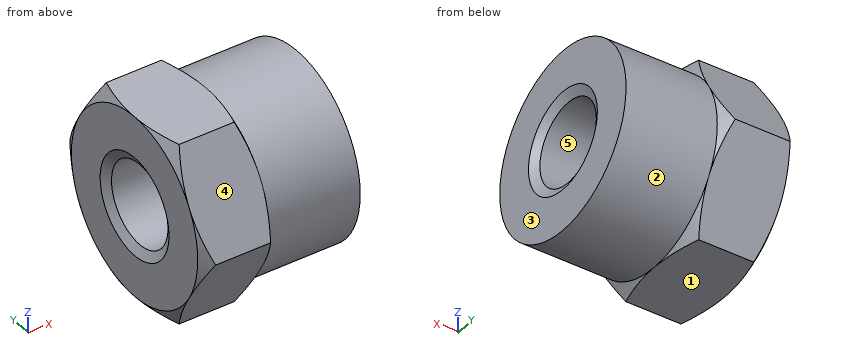
Autodesk Inventor part; units mm, degrees
ref_plane "Work Plane1" through (9.7259, 0, 0) normal (0, 0, 1) x (-1, 0, 0)
ref_plane "YZ Plane" through (0, 0, 0) normal (1, 0, 0) x (0, 1, 0)
ref_plane "XZ Plane" through (0, 0, 0) normal (0, 1, 0) x (-1, 0, 0)
sketch "Sketch1" plane through (0, 0, 0) normal (1, 0, 0) x (0, 1, 0)
  line L0 (1.5877, -2.75) -> (-1.5877, -2.75)
  line L1 (-1.5877, -2.75) -> (-3.1754, 0)
  line L2 (-3.1754, 0) -> (-1.5877, 2.75)
  line L3 (-1.5877, 2.75) -> (1.5877, 2.75)
  line L4 (1.5877, 2.75) -> (3.1754, 0)
  line L5 (3.1754, 0) -> (1.5877, -2.75)
  point P0 (0, 0)
  point P1 (0, 0)
  dimension "d0" = 6.3509
extrude "Body" add sketch "Sketch1" along normal blind 2.15
sketch "Sketch2" plane through (2.15, 0, 0) normal (1, 0, 0) x (0, 0, -1)
  circle A0 centre (0, 0) radius 2.75
  dimension "d7" = 5.5
extrude "Ring" add sketch "Sketch2" along normal blind 2.75
sketch "Sketch3" plane through (0, 0, 0) normal (0, 0, 1) x (1, 0, 0)
  line L0 (0, 1.5877) -> (0, 3.1754)
  line L1 (0, 3.1754) -> (2.15, 3.1754)
  line L2 (2.15, 1.5877) -> (2.15, 3.1754)
  line L3 (-0.43, 0) -> (2.58, 0)
  line L4 (0, 2.75) -> (0.2456, 3.1754)
  line L5 (1.9044, 3.1754) -> (2.15, 2.75)
  dimension "d3" = 30
  dimension "d4" = 30
  dimension "d5" = 5.5
  dimension "d6" = 5.5
revolve "Chamfer1" cut sketch "Sketch3" angle 360 about axis through (-10, 0, 0) along (1, 0, 0)
sketch "Sketch4" plane through (0, 0, 0) normal (-1, 0, 0) x (0, 0, 1)
  line L0 (0, -4.4456) -> (0, 4.4456)
  line L1 (-3.85, 0) -> (3.85, 0)
  point P0 (0, 0)
hole "Thread" at (0, 0, 0) direction (1, 0, 0) diameter 2.459 end through all
chamfer "Chamfer2" distance 0.2706 angle 30 1 edges at (0, 0, -1.2295) measured on face at (0, -2.2301, 0.0494)
chamfer "Chamfer3" distance 0.2706 angle 30 1 edges at (4.9, 0, -1.2295) measured on face at (4.9, -0.3175, -2.2046)
ref_plane "Work Plane1" through (9.7259, 0, 0) normal (0, 0, 1) x (-1, 0, 0)
equation "\"d0\" = 1.1547 * SW"
equation "\"d1\" = KOH1"
equation "\"d7\" = SD2"
equation "\"d8\" = KOH - KOH1"
equation "\"d3\" = ANG1"
equation "\"d4\" = ANG2"
equation "\"d5\" = SW0"
equation "\"d6\" = SW01"
equation "\"d10\" = -0.5 * GD1 + 0.5 * NND"
equation "\"d46\" = -0.5 * GD1 + 0.5 * NND"
equation "\"d12\" = -0.5 * GD1 + 0.5 * NND"
equation "\"d47\" = -0.5 * GD1 + 0.5 * NND"
equation "\"ANG1\" = 30deg"
equation "\"ANG2\" = ANG1"
equation "\"NND\" = 3"
equation "\"KOH1\" = 2.15"
equation "\"KOH\" = 4.9"
equation "\"SW\" = 5.5"
equation "\"SW0\" = SW"
equation "\"SW01\" = SW"
equation "\"SD2\" = SW"
equation "\"GUL\" = 0.541266 * PTC"
equation "\"THREADDIA\" = 3"
equation "\"TOA\" = 30deg"
equation "\"PTC\" = 0.5"
equation "\"E0\" = 1.155 * SW"
equation "\"GAL\" = 0.541266 * PTC"
properties part number "NF E 25-409 - M3" material "Steel, Mild"
Geometry check sheet. Reference: the model listing, model coordinates, mm. Face numbers are marked on the shaded views. A direction names the side the tool comes from. Give positions to 0.01 mm unless a question says otherwise; leave off trailing zeros. Write each loop counter-clockwise with the first axis right and the second up, starting at its lowest first coordinate (ties: lowest second). Pieces come first, ordered by that corner, then holes. Notation, with made-up numbers: (-15.75, 82.25) -> (27.25, 82.25) arc R34 ccw to (27.25, 115.25) -> close; hole circle Ø2 at (54.5, 89). An arc over 180 degrees is marked (long way). Use one line per item in the form item = value.
Item 1: Sectioned sample at B-B on x = 2.9. Enter the section's corners in (y, z).
Results list:
outline = circle Ø5.5 at (0, 0); hole circle Ø2.46 at (0, 0)
Item 2: Access from +Z, -Z, +X, -X, +Y, -Y to the whole of each face (thin tool, end or side, straight path). Record for the marked faces 1 and 2.
Results list:
face_1 = -Z, +X, -X, +Y, -Y
face_2 = +X
Item 3: Scan line: line 1 (Z direction, x = 1.65, y = 0). Record every from-to range of solid material in increasing order.
Results list:
line_1 = -2.75 to -1.23, 1.23 to 2.75
Item 4: Depth check by flat-ended pin: pin 1 Ø2 at (x, z) = (3, 1) entering from +Y; pin 2 Ø2 at (y, z) = (0, 0) entering from +X. Enter the tip coordinate at first touch or a pass-through.
Results list:
pin_1 = 2.81
pin_2 = through
Item 5: Mould release check, pull along Y, two halves, no side actions. Record for the marked faces 3, 4 and 5: released by +Y, released by -Y, zero draft, split by the parting line, or undercut.
Results list:
face_3 = zero draft
face_4 = released by -Y
face_5 = undercut
Item 6: Sectioned sample at A-A on x = 1.65. Enter the section's corners in (y, z), plus the area to 3 significant figures.
Results list:
outline = (-3.18, 0) -> (-1.59, -2.75) -> (1.59, -2.75) -> (3.18, 0) -> (1.59, 2.75) -> (-1.59, 2.75) -> close; hole circle Ø2.46 at (0, 0)
area = 21.4 mm2
